CAD build for the part. Positions are in the model's coordinates, mm. A direction names the side the tool comes from. Round coordinates to 2 decimals unless told otherwise and drop trailing zeros. Loops run counter-clockwise (first coordinate to the right, second up) from the corner with the lowest first, then second, coordinate; pieces in that order, holes last. Notation, with made-up numbers: (-4.75, 44) - (8.25, 44) arc R19 cw to (8.25, 77) - close; hole circle Ø2 at (-32.5, -22.75). An arc over 180 degrees is marked (long way). Use one line per item in the form item = value.
from build123d import *

# Parameters (mm, degrees)
SKETCH_1_R      = 1
SKETCH_1_R_2    = 1.025
SKETCH_1_W      = 20.3
SKETCH_1_H      = 8.6
SKETCH_1_W_2    = 1.5
SKETCH_1_H_2    = 4
EXTRUDE_1_DEPTH = 1.5
FILLET_1_R      = 1


with BuildPart() as part:
    # 草图1 → 凸台-拉伸1 (new body)
    with BuildSketch(Plane.XY):
        Polygon((-16.136931804, -26.136931804), (-16.136931804, 14.136931804), (-6.414578713, 14.136931804), (-6.414578713, 44.863068196), (-16.136931804, 44.863068196), (-16.136931804, 53.863068196), (-11.136931804, 53.863068196), (-11.136931804, 50.363068196), (-11.786931804, 50.363068196), (-11.786931804, 48.863068196), (-7.386931804, 48.863068196), (-7.386931804, 50.363068196), (-9.586931804, 50.363068196), (-9.586931804, 53.863068196), (-4.586931804, 53.863068196), (-4.586931804, 48.863068196), (45.413068196, 48.863068196), (45.413068196, 53.863068196), (50.413068196, 53.863068196), (50.413068196, 50.363068196), (48.213068196, 50.363068196), (48.213068196, 48.863068196), (50.413068196, 48.863068196), (51.913068196, 48.863068196), (52.613068196, 48.863068196), (52.613068196, 50.363068196), (51.913068196, 50.363068196), (51.913068196, 53.863068196), (56.913068196, 53.863068196), (56.913068196, 23.363068196), (27.29285372, 23.363068196), (17.863068196, 11.732999384), (17.863068196, -6.588407425), (23.863068196, -6.588407425), (23.863068196, -12.588407425), (17.863068196, -12.588407425), (17.863068196, -26.136931804), align=None)
        with Locations((11.136931804, 11.136931804)):
            Circle(SKETCH_1_R, mode=Mode.SUBTRACT)
        with Locations((31, 30)):
            Circle(SKETCH_1_R, mode=Mode.SUBTRACT)
        with Locations((54.5, 30)):
            Circle(SKETCH_1_R, mode=Mode.SUBTRACT)
        with Locations((20.863068196, -9.588407425)):
            Circle(SKETCH_1_R_2, mode=Mode.SUBTRACT)
        with Locations((25.863068196, 26.363068196)):
            Circle(SKETCH_1_R, mode=Mode.SUBTRACT)
        with Locations((40.863068196, 44.863068196)):
            Circle(SKETCH_1_R, mode=Mode.SUBTRACT)
        with Locations((10.863068196, 44.863068196)):
            Circle(SKETCH_1_R, mode=Mode.SUBTRACT)
        with Locations((51.138068196, 38.863068196)):
            Circle(SKETCH_1_R, mode=Mode.SUBTRACT)
        with Locations((11.136931804, -11.136931804)):
            Circle(SKETCH_1_R, mode=Mode.SUBTRACT)
        with Locations((-11.136931804, -11.136931804)):
            Circle(SKETCH_1_R, mode=Mode.SUBTRACT)
        with Locations((-11.136931804, 11.136931804)):
            Circle(SKETCH_1_R, mode=Mode.SUBTRACT)
        with Locations((42.75, 30)):
            Rectangle(SKETCH_1_W, SKETCH_1_H, mode=Mode.SUBTRACT)
        with Locations((-9.636931804, -22.636931804)):
            Rectangle(SKETCH_1_W_2, SKETCH_1_H_2, mode=Mode.SUBTRACT)
        with Locations((14.863068196, -22.636931804)):
            Rectangle(SKETCH_1_W_2, SKETCH_1_H_2, mode=Mode.SUBTRACT)
        with Locations((12.363068196, -22.636931804)):
            Rectangle(SKETCH_1_W_2, SKETCH_1_H_2, mode=Mode.SUBTRACT)
        with Locations((-13.136931804, -22.636931804)):
            Rectangle(SKETCH_1_W_2, SKETCH_1_H_2, mode=Mode.SUBTRACT)
        Polygon((37.00085024, 44.863068196), (14.725286152, 44.863068196), (25.863068196, 31.126470342), align=None, mode=Mode.SUBTRACT)
        with Locations((9.863068196, -22.636931804)):
            Rectangle(SKETCH_1_W_2, SKETCH_1_H_2, mode=Mode.SUBTRACT)
        with Locations((7.363068196, -22.636931804)):
            Rectangle(SKETCH_1_W_2, SKETCH_1_H_2, mode=Mode.SUBTRACT)
        with Locations((4.863068196, -22.636931804)):
            Rectangle(SKETCH_1_W_2, SKETCH_1_H_2, mode=Mode.SUBTRACT)
        with Locations((2.363068196, -22.636931804)):
            Rectangle(SKETCH_1_W_2, SKETCH_1_H_2, mode=Mode.SUBTRACT)
        with Locations((-0.136931804, -22.636931804)):
            Rectangle(SKETCH_1_W_2, SKETCH_1_H_2, mode=Mode.SUBTRACT)
        with Locations((-2.636931804, -22.636931804)):
            Rectangle(SKETCH_1_W_2, SKETCH_1_H_2, mode=Mode.SUBTRACT)
        with Locations((-5.136931804, -22.636931804)):
            Rectangle(SKETCH_1_W_2, SKETCH_1_H_2, mode=Mode.SUBTRACT)
        Polygon((-11.136931804, 0), (0, 11.136931804), (11.136931804, 0), (0, -11.136931804), align=None, mode=Mode.SUBTRACT)
        Polygon((22.00085024, 26.363068196), (12.087766679, 14.136931804), (-0.414578713, 14.136931804), (-0.414578713, 44.863068196), (7.00085024, 44.863068196), align=None, mode=Mode.SUBTRACT)
        Polygon((38.430635764, 41.863068196), (34.73085074, 37.3), (36.73085074, 37.3), (40.430635764, 41.863068196), align=None, mode=Mode.SUBTRACT)
        Polygon((43.430635764, 41.863068196), (39.73085074, 37.3), (41.73085074, 37.3), (45.430635764, 41.863068196), align=None, mode=Mode.SUBTRACT)
        Polygon((48.430635764, 41.863068196), (44.73085074, 37.3), (46.73085074, 37.3), (50.430635764, 41.863068196), align=None, mode=Mode.SUBTRACT)
        Polygon((-8.43714678, -14.136931804), (-12.136931804, -18.7), (-10.136931804, -18.7), (-6.43714678, -14.136931804), align=None, mode=Mode.SUBTRACT)
        Polygon((-3.43714678, -14.136931804), (-7.136931804, -18.7), (-5.136931804, -18.7), (-1.43714678, -14.136931804), align=None, mode=Mode.SUBTRACT)
        Polygon((1.56285322, -14.136931804), (-2.136931804, -18.7), (-0.136931804, -18.7), (3.56285322, -14.136931804), align=None, mode=Mode.SUBTRACT)
        Polygon((6.56285322, -14.136931804), (2.863068196, -18.7), (4.863068196, -18.7), (8.56285322, -14.136931804), align=None, mode=Mode.SUBTRACT)
        Polygon((11.56285322, -14.136931804), (7.863068196, -18.7), (9.863068196, -18.7), (13.56285322, -14.136931804), align=None, mode=Mode.SUBTRACT)
    extrude(amount=EXTRUDE_1_DEPTH)

    # 圆角1
    fillet_1_edges = [part.edges().sort_by_distance(p)[0] for p in [
        (-16.136931804, -26.136931804, 0.75),
        (-16.136931804, 14.136931804, 0.75),
        (-16.136931804, 44.863068196, 0.75),
        (-16.136931804, 53.863068196, 0.75),
        (-4.586931804, 53.863068196, 0.75),
        (45.413068196, 53.863068196, 0.75),
        (56.913068196, 53.863068196, 0.75),
        (56.913068196, 23.363068196, 0.75),
        (23.863068196, -6.588407425, 0.75),
        (23.863068196, -12.588407425, 0.75),
        (17.863068196, -26.136931804, 0.75),
    ]]
    fillet(fillet_1_edges, radius=FILLET_1_R)


solid = part.part
1) Slice it at A-A (x = 54.5). Write the cut outline in (y, z).
Report:
outline = (23.36, 0) - (29, 0) - (29, 1.5) - (23.36, 1.5) - close; (31, 0) - (53.86, 0) - (53.86, 1.5) - (31, 1.5) - close
2) Tool access for faces 1 (the flat face through (12.4, 14, 1.5)), 2 (the flat face through (1.687, -16.45, 0.74)): list every direction of +Z, -Z, +X, -X, +Y, -Y with a clear straight run to the whole face (end or side of a thin tool).
Report:
face_1 = +Z, +X, -X, +Y, -Y
face_2 = +Z, -Z
3) Drill centre lines: probe 1 along Y at (x, z) = (33.5, 1.2); probe 2 along Y at (x, z) = (18.5, 1.1); probe 3 along Y at (x, z) = (51, 0.2). Where is each one in solid material? Low to high.
Report:
probe_1 = 23.36 to 25.7, 34.3 to 40.55, 44.86 to 48.86
probe_2 = -12.59 to -6.59, 12.52 to 22.05, 30.68 to 40.21, 44.86 to 48.86
probe_3 = 23.36 to 25.7, 34.3 to 37.87, 39.85 to 48.86
4) Slice it at D-D (y = 9). Write the cut outline in (x, z).
Report:
outline = (-16.14, 0) - (-2.14, 0) - (-2.14, 1.5) - (-16.14, 1.5) - close; (2.14, 0) - (17.86, 0) - (17.86, 1.5) - (2.14, 1.5) - close
5) Slice it at B-B (y = 30). Write the cut outline in (x, z).
Report:
outline = (-6.41, 0) - (-0.41, 0) - (-0.41, 1.5) - (-6.41, 1.5) - close; (19.05, 0) - (30, 0) - (30, 1.5) - (19.05, 1.5) - close; (32, 0) - (32.6, 0) - (32.6, 1.5) - (32, 1.5) - close; (52.9, 0) - (53.5, 0) - (53.5, 1.5) - (52.9, 1.5) - close; (55.5, 0) - (56.91, 0) - (56.91, 1.5) - (55.5, 1.5) - close
6) Flat gauge pin, fed straight in: pin 1 (1.8 mm diameter, centred on x = 10.86, y = 44.86, fed in from -Z). Where does the tip first touch, or does it go through?
Report:
pin_1 = through
7) Slice it at C-C (x = 31). Write the cut outline in (y, z), plus the area to 3 significant figures.
Report:
outline = (23.36, 0) - (29, 0) - (29, 1.5) - (23.36, 1.5) - close; (31, 0) - (37.46, 0) - (37.46, 1.5) - (31, 1.5) - close; (44.86, 0) - (48.86, 0) - (48.86, 1.5) - (44.86, 1.5) - close
area = 24.1 mm^2
8) Two-plate mould, pull along Y, no slides. Class faces 3 (the flat face through (12.4, 14, 0)), 4 (the flat face through (4.739, -16.387, 0.74)), 5 (the cylindrical face through (12.1, 11.4, 0.7)): +Y half, -Y half, draft (parallel to the pull), parting line (faces both ways), or undercut.
Report:
face_3 = draft
face_4 = undercut
face_5 = undercut
